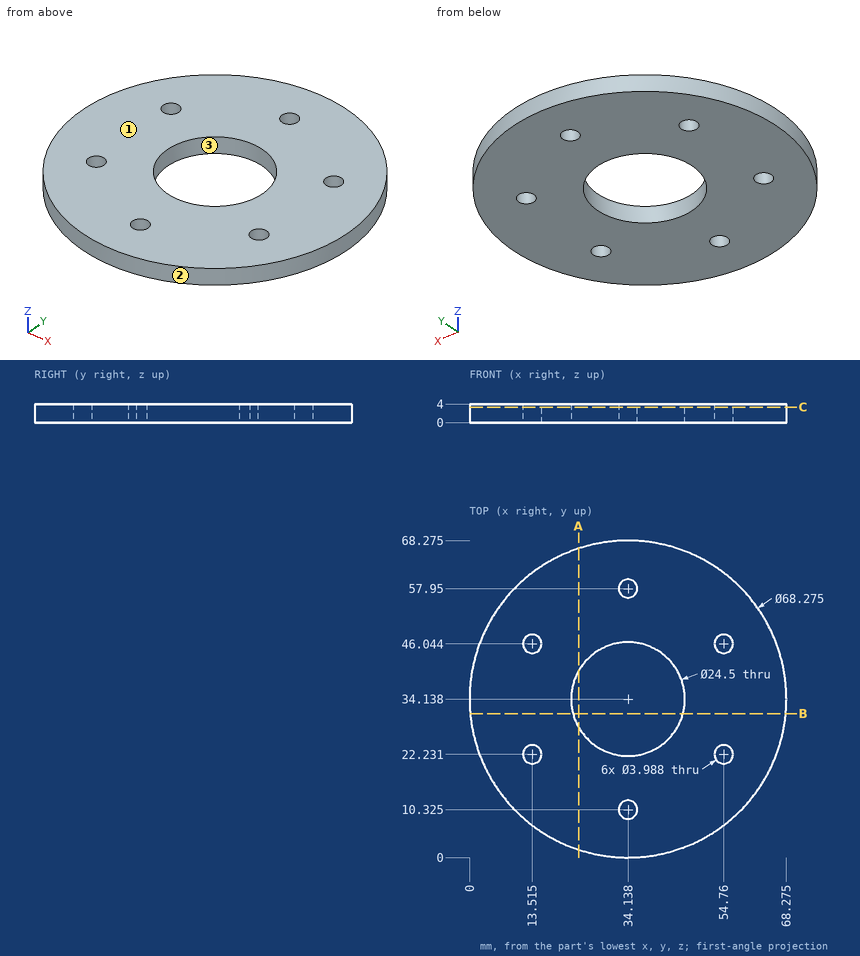
Study the drawing (mm; zero at the part's minimum x, y, z) and answer. Round coordinates to 2 decimals unless told otherwise and drop trailing zeros. Write each loop counter-clockwise with the first axis right and the second up, starting at its lowest first coordinate (ties: lowest second). Pieces come first, ordered by that corner, then holes. Notation, with made-up numbers: (45, 88) - (76, 88) arc R34 cw to (76, 118) - close; hole circle Ø1 at (23, 4.5). An arc over 180 degrees is marked (long way). Use a Markdown table: item, result. Add a question column.
1. The part is cut by section B-B (y = 31). Write down the section's boundary in (x, z) (1 decimal), and give its area (3 significant figures).
2. Consider line 1 (Y direction, x = 54.5, z = 3.25) (1 decimal); line 2 (X direction, y = 47, z = 3.25) (1 decimal); line 3 (Y direction, x = 53, z = 3.8) (1 decimal). Determine where each line is inside the solid, lowest interval first.
3. For a pull along Y with two mould halves and no side action, classify the marked faces 1, 2 and 3 as +Y half, -Y half, draft (parallel to the pull), parting line (faces both ways), or undercut.
4. The part is cut by section C-C (z = 3.3). Give the number of separate pieces and of enclosed holes in the cut face.
5. A flat-ended cylindrical pin translates along its axis: P1, Ø1, axis at x = 56, z = 2.5, coming from the +Y side (1 decimal). Find the tip coordinate at first contact, or state that the pin passes through.
6. The part is cut by section A-A (x = 23.5). Write down the section's boundary in (y, z) (1 decimal).
Reported:
| question | item | result |
|---|---|---|
| 1 | outline | (0.1, 0) - (22.3, 0) - (22.3, 4) - (0.1, 4) - close; (46, 0) - (68.1, 0) - (68.1, 4) - (46, 4) - close |
| 1 | area | 177 mm^2 |
| 2 | line 1 | 6.7 to 20.3, 24.2 to 44.1, 48 to 61.5 |
| 2 | line 2 | 2.5 to 11.8, 15.3 to 53, 56.5 to 65.8 |
| 2 | line 3 | 5.7 to 21.3, 23.2 to 45.1, 47 to 62.6 |
| 3 | face 1 | draft |
| 3 | face 2 | parting line |
| 3 | face 3 | undercut |
| 4 | separate pieces | 1 |
| 4 | enclosed holes | 7 |
| 5 | P1 | y = 60.8 |
| 6 | outline | (1.7, 0) - (28.1, 0) - (28.1, 4) - (1.7, 4) - close; (40.2, 0) - (66.6, 0) - (66.6, 4) - (40.2, 4) - close |
